Part model, mm, in its own coordinate system. A direction names the side the tool comes from. Round coordinates to 2 decimals unless told otherwise and drop trailing zeros. Loops run counter-clockwise (first coordinate to the right, second up) from the corner with the lowest first, then second, coordinate; pieces in that order, holes last. Notation, with made-up numbers: (-26.5, 88) -> (6.5, 88) arc R19 cw to (6.5, 112) -> close; hole circle Ø11 at (-12.5, -27.75). An arc over 180 degrees is marked (long way). Use a Markdown table: item, result. Add a question column.
Item 1: Flat gauge pins, fed straight in: pin 1 (10 mm diameter, centred on x = -3.5, y = -9, fed in from +Z); pin 2 (1.4 mm diameter, centred on x = 0.5, y = 1, fed in from +Z). Where does each tip first touch, or does it go through?
Item 2: Two-plate mould, pull along X, no slides. Class faces 3 (the face through (3, 0, 0)), 4 (the face through (0, 0, 0.5)), 5 (the face through (-2.8, 0.1, 1.5)): pulls with the +X half, pulls with the -X half, needs draft (parallel to the pull), parting line crosses it, or undercut.
Item 3: Cut at D-D, the plane z = -0.5. List the corners of the cut face in (x, y), plus the area to 3 significant figures.
Item 4: Which spindle directions (+Z, -Z, +X, -X, +Y, -Y) get a long thin tool onto all of the face, cutting with end or side? Do faces 1 (the face through (-1.825, -1.4, 1.979)), 2 (the face through (0, 0, -2)). Say none if no direction does.
Item 5: Probe line 1 (Y direction, x = 0, z = 1.9); line 2 (X direction, y = 1.25, z = 1.45); line 3 (Z direction, x = -4.75, y = -4). List the from-to ranges inside material, lowest first. Write a range as [from, to].
Item 6: Cut at C-C, the plane z = 1.2. List the corners of the cut face in (x, y).
```python
from build123d import *

# Parameters (mm, degrees)
F0_R      = 2.8
F1_DEPTH  = 3.5
F2_T      = -0.5
F0_R_2    = 15
F1_FACE_R = 2.8
F3_DEPTH  = 2
F4_R      = 1.99999
F5_SIZE   = 0.4


# Not quite as in the source:
# - a fillet or chamfer is up to 0.001 mm smaller than in the source, because OpenCascade refuses the exact size


with BuildPart() as f1:
    # F0 (on Top) → F1 (new body)
    with BuildSketch(Plane.XY):
        Circle(F0_R)
    extrude(amount=F1_DEPTH)

    # F2
    f2_openings = [f1.faces().sort_by_distance(p)[0] for p in [
        (0, 0, 3.5),
    ]]
    offset(amount=F2_T, openings=f2_openings)

    # F0 (on Top) + F1_face (on face) → F3 (join)
    with BuildSketch(Plane.XY):
        Circle(F0_R_2)
        Circle(F0_R, mode=Mode.SUBTRACT)
    with BuildSketch(Plane(origin=(0, 0, 0), x_dir=(1, 0, 0), z_dir=(0, 0, -1))):
        Circle(F1_FACE_R)
    extrude(amount=-F3_DEPTH, dir=(0, 0, 1))

    # F4 (radius 2 in the source; OpenCascade refuses exactly that, so slightly less here)
    f4_edges = [f1.edges().sort_by_distance(p)[0] for p in [
        (-15, 0, -2),
    ]]
    fillet(f4_edges, radius=F4_R)

    # F5
    f5_edges = [f1.edges().sort_by_distance(p)[0] for p in [
        (-2.8, 0, 3.5),
    ]]
    chamfer(f5_edges, length=F5_SIZE)


solid = f1.part
```
A:
| question | item | result |
|---|---|---|
| 1 | pin 1 | stops at z = 0 |
| 1 | pin 2 | stops at z = 0.5 |
| 2 | face 3 | needs draft |
| 2 | face 4 | undercut |
| 2 | face 5 | parting line crosses it |
| 3 | outline | circle Ø29.87 at (0, 0) |
| 3 | area | 701 mm^2 |
| 4 | face 1 | +Z |
| 4 | face 2 | -Z, +X, -X, +Y, -Y |
| 5 | line 1 | y = [-2.8, -2.3], [2.3, 2.8] |
| 5 | line 2 | x = [-2.51, -1.93], [1.93, 2.51] |
| 5 | line 3 | z = [-2, 0] |
| 6 | outline | circle Ø5.6 at (0, 0); hole circle Ø4.6 at (0, 0) |
